The model under review builds one solid part; all positions refer to its coordinate system, in mm. A direction names the side the tool comes from. Give positions to 0.01 mm unless a question says otherwise; leave off trailing zeros. Order: outer loops, then holes, each group sorted by start corner. A loop starts at its lowest first (then second) coordinate and runs counter-clockwise, first axis right, second up.
```python
from build123d import *

# Parameters (mm, degrees)
SKETCH1_W                    = 114.3
SKETCH1_H                    = 78.232
BOSS_EXTRUDE1_DEPTH          = 3.175
EDGE_FLANGE1_STRIP_W         = 14.224
EDGE_FLANGE1_STRIP_H         = 3.175
EDGE_FLANGE1_STRIP_CUT_DEPTH = 114.3
EDGE_FLANGE1_DEPTH           = 114.3
EDGE_FLANGE2_STRIP_W         = 14.224
EDGE_FLANGE2_STRIP_H         = 3.175
EDGE_FLANGE2_STRIP_CUT_DEPTH = 114.3
EDGE_FLANGE2_DEPTH           = 114.3
SKETCH9_R                    = 2.667
CUT_EXTRUDE1_DEPTH           = 145.648316869
CHAMFER1_SIZE                = 3.175
SKETCH15_W                   = 114.3
SKETCH15_H                   = 36.5125
BOSS_EXTRUDE2_DEPTH          = 3.175
SKETCH16_W                   = 114.3
SKETCH16_H                   = 50.8
BOSS_EXTRUDE3_DEPTH          = 3.175


# Sheet-metal steps are written as plain solids
with BuildPart() as part:
    # Sketch1 → Boss-Extrude1 (new body)
    with BuildSketch(Plane(origin=(0, 0, 0), x_dir=(1, 0, 0), z_dir=(0, 1, 0))):
        with Locations((57.15, 39.116)):
            Rectangle(SKETCH1_W, SKETCH1_H)
    extrude(amount=BOSS_EXTRUDE1_DEPTH)

    # Edge-Flange1 strip (across the edge) → Edge-Flange1 strip cut (cut)
    with BuildSketch(Plane(origin=(114.3, 3.175, -78.232), x_dir=(0, 0, 1), z_dir=(-1, 0, 0))):
        with Locations((-6.35, -1.5875)):
            Rectangle(EDGE_FLANGE1_STRIP_W, EDGE_FLANGE1_STRIP_H)
    extrude(amount=EDGE_FLANGE1_STRIP_CUT_DEPTH, mode=Mode.SUBTRACT)

    # Edge-Flange1 section (across the edge) → Edge-Flange1 (add)
    with BuildSketch(Plane(origin=(114.3, 3.175, -78.232), x_dir=(0, 0, 1), z_dir=(-1, 0, 0))):
        with BuildLine():
            Line((-3.175, 0.762), (-3.175, 23.368))
            Line((-3.175, 23.368), (0, 23.368))
            Line((0, 23.368), (0, 0.762))
            ThreePointArc((0, 0.762), (0.223184633, 0.223184633), (0.762, 0))
            Line((0.762, 0), (0.762, -3.175))
            ThreePointArc((0.762, -3.175), (-2.021879398, -2.021879398), (-3.175, 0.762))
        make_face()
    extrude(amount=EDGE_FLANGE1_DEPTH)

    # Edge-Flange2 strip (across the edge) → Edge-Flange2 strip cut (cut)
    with BuildSketch(Plane(origin=(0, 3.175, 0), x_dir=(0, 0, -1), z_dir=(1, 0, 0))):
        with Locations((-6.35, -1.5875)):
            Rectangle(EDGE_FLANGE2_STRIP_W, EDGE_FLANGE2_STRIP_H)
    extrude(amount=EDGE_FLANGE2_STRIP_CUT_DEPTH, mode=Mode.SUBTRACT)

    # Edge-Flange2 section (across the edge) → Edge-Flange2 (add)
    with BuildSketch(Plane(origin=(0, 3.175, 0), x_dir=(0, 0, -1), z_dir=(1, 0, 0))):
        with BuildLine():
            Line((-3.175, 0.762), (-3.175, 23.368))
            Line((-3.175, 23.368), (0, 23.368))
            Line((0, 23.368), (0, 0.762))
            ThreePointArc((0, 0.762), (0.223184633, 0.223184633), (0.762, 0))
            Line((0.762, 0), (0.762, -3.175))
            ThreePointArc((0.762, -3.175), (-2.021879398, -2.021879398), (-3.175, 0.762))
        make_face()
    extrude(amount=EDGE_FLANGE2_DEPTH)

    # Sketch9 → Cut-Extrude1 (cut, through all)
    with BuildSketch(Plane.XY.offset(3.175)):
        with Locations((107.95, 16.637)):
            Circle(SKETCH9_R)
    extrude(amount=-CUT_EXTRUDE1_DEPTH, mode=Mode.SUBTRACT)

    # Chamfer1
    chamfer1_edges = [part.edges().sort_by_distance(p)[0] for p in [
        (114.3, 26.543, -79.8195),
        (0, 26.543, -79.8195),
        (0, 26.543, 1.5875),
        (114.3, 26.543, 1.5875),
    ]]
    chamfer(chamfer1_edges, length=CHAMFER1_SIZE)

    # Sketch15 → Boss-Extrude2 (add)
    with BuildSketch(Plane.XY.offset(3.175)):
        with Locations((57.15, 18.25625)):
            Rectangle(SKETCH15_W, SKETCH15_H)
    extrude(amount=-BOSS_EXTRUDE2_DEPTH)

    # Sketch16 → Boss-Extrude3 (add)
    with BuildSketch(Plane(origin=(0, 0, -81.407), x_dir=(-1, 0, 0), z_dir=(0, 0, -1))):
        with Locations((-57.15, 25.4)):
            Rectangle(SKETCH16_W, SKETCH16_H)
    extrude(amount=-BOSS_EXTRUDE3_DEPTH)


solid = part.part
```
1. Insertion check: pin 1 (4 mm diameter, centred on x = 96, z = -8, fed in from +Y) (3 decimals); pin 2 (2.5 mm diameter, centred on x = 56, z = 1.5, fed in from +Y). Each pin has a flat end and moves straight along its axis. Give the tip position at first contact, or say it passes through.
2. To check wall thickness, follow line 1 (Z direction, x = 100, y = 25.5) (3 decimals); line 2 (Y direction, x = 86, z = -77.5); line 3 (Z direction, x = 19.5, y = 38.5). State the ranges of each line that lie inside material, in increasing order.
3. Draft analysis for pull direction Z (two halves, no side actions). For faces 3 (the flat face through (58, 28, -78.232)), 4 (the flat face through (56, 3.175, -40)), 5 (the flat face through (56, 19, 3.175)), 6 (the flat face through (56, 36.512, 2)), state which applies: pulls with the +Z half, pulls with the -Z half, needs draft (parallel to the pull), parting line crosses it, or undercut.
4. Take a section at C-C (y = 38). Write out the cut boundary in (x, z), and give its area (3 significant figures).
5. Take a section at D-D (z = -2.5). Write out the cut boundary in (x, y) (3 decimals), and give its area (3 significant figures).
6. For faces 1 (the flat face through (114.3, 3, -42)), 2 (the flat face through (56, 20, 0)), list the 3-axis set-ups (+Z, -Z, +X, -X, +Y, -Y) from which the entire face can be reached by the end or side of a thin tool; tool diameter is ignored.
7. Take a section at A-A (y = 12). Write out the cut boundary in (x, z) (3 decimals).
Answer:
1. pin 1: stops at y = 3.175
1. pin 2: stops at y = 36.51
2. line 1: z = -81.407 to -78.232, 0 to 3.175
2. line 2: y = 0 to 3.18
2. line 3: z = -81.41 to -78.23
3. face 3: undercut
3. face 4: undercut
3. face 5: pulls with the +Z half
3. face 6: needs draft
4. outline: (0, -81.41) - (114.3, -81.41) - (114.3, -78.23) - (0, -78.23) - close
4. area: 363 mm2
5. outline: (0, 0) - (114.3, 0) - (114.3, 3.175) - (0, 3.175) - close
5. area: 363 mm2
6. face 1: +Z, -Z, +X, +Y, -Y
6. face 2: +X, -X, +Y
7. outline: (0, -81.407) - (114.3, -81.407) - (114.3, -78.232) - (0, -78.232) - close; (0, 0) - (114.3, 0) - (114.3, 3.175) - (0, 3.175) - close
